Autodesk Inventor part; units mm, degrees
ref_plane "YZ Plane" through (0, 0, 0) normal (1, 0, 0) x (0, 1, 0)
ref_plane "XZ Plane" through (0, 0, 0) normal (0, 1, 0) x (-1, 0, 0)
ref_plane "XY Plane" through (0, 0, 0) normal (0, 0, 1) x (1, 0, 0)
ref_plane "Work Plane1" through (0, 0, 0) normal (0, 0, 1) x (1, 0, 0)
sketch "Sketch1" plane through (0, 0, 0) normal (0, 0, 1) x (1, 0, 0)
  circle A0 centre (11.7233, 46.6483) radius 2.132
  circle A1 centre (20.0025, 56.1975) radius 2.132
  circle A2 centre (32.7025, 56.1975) radius 2.132
  circle A3 centre (45.4025, 56.1975) radius 2.132
  circle A4 centre (58.1025, 56.1975) radius 2.132
  circle A5 centre (-58.7375, 17.4625) radius 2.132
  circle A6 centre (-46.6483, 46.6483) radius 2.132
  circle A7 centre (-17.4625, 58.7375) radius 2.132
  circle A8 centre (11.7233, 46.6483) radius 2.132
  circle A9 centre (23.8125, 17.4625) radius 2.132
  circle A10 centre (11.7233, -11.7233) radius 2.132
  circle A11 centre (-17.4625, -23.8125) radius 2.132
  circle A12 centre (-46.6483, -11.7233) radius 2.132
  circle A13 centre (-56.1975, -32.7025) radius 2.132
  circle A14 centre (-56.1975, -45.4025) radius 2.132
  circle A15 centre (-56.1975, -58.1025) radius 2.132
  circle A16 centre (-56.1975, -20.0025) radius 2.132
  circle A17 centre (-17.4625, 17.4625) radius 38.1
  circle A18 centre (-17.4625, 17.4625) radius 38.3
  circle A19 centre (-17.4625, 17.4625) radius 45.72
  circle A20 centre (-17.4625, 17.4625) radius 32.55
  line L0 (9.485, -18.7266) -> (-48.7269, -62.0728)
  arc A21 (9.485, -18.7266) -> (18.7266, -9.485) centre (-17.4625, 17.4625) ccw
  line L1 (62.0728, 48.7269) -> (18.7266, -9.485)
  arc A22 (62.0728, 48.7269) -> (62.5825, 50.2648) centre (60.0075, 50.2648) ccw
  line L2 (62.5825, 60.0075) -> (62.5825, 50.2648)
  arc A23 (62.5825, 60.0075) -> (60.0075, 62.5825) centre (60.0075, 60.0075) ccw
  line L3 (-17.4625, 62.5825) -> (60.0075, 62.5825)
  arc A24 (-17.4625, 62.5825) -> (-62.5825, 17.4625) centre (-17.4625, 17.4625) ccw
  line L4 (-62.5825, -60.0075) -> (-62.5825, 17.4625)
  arc A25 (-62.5825, -60.0075) -> (-60.0075, -62.5825) centre (-60.0075, -60.0075) ccw
  line L5 (-50.2648, -62.5825) -> (-60.0075, -62.5825)
  arc A26 (-50.2648, -62.5825) -> (-48.7269, -62.0728) centre (-50.2648, -60.0075) ccw
  arc A27 (-46.4955, -21.6632) -> (-38.635, -17.6063) centre (-46.6483, -11.7233) ccw
  arc A28 (-33.9418, -16.445) -> (-38.635, -17.6063) centre (-35.592, -19.8403) ccw
  arc A29 (-33.9418, -16.445) -> (-29.7861, -18.1664) centre (-17.4625, 17.4625) ccw
  arc A30 (-27.2887, -22.3061) -> (-29.7861, -18.1664) centre (-31.0201, -21.734) ccw
  arc A31 (-27.2887, -22.3061) -> (-26.8535, -27.0731) centre (-17.4625, -23.8125) ccw
  arc A32 (-28.1651, -31.3391) -> (-26.8535, -27.0731) centre (-30.4197, -28.3113) ccw
  line L6 (-44.1828, -43.2664) -> (-28.1651, -31.3391)
  arc A33 (-50.2124, -40.2386) -> (-44.1828, -43.2664) centre (-46.4374, -40.2386) ccw
  line L7 (-50.2124, -25.4377) -> (-50.2124, -40.2386)
  arc A34 (-46.4955, -21.6632) -> (-50.2124, -25.4377) centre (-46.4374, -25.4377) ccw
  line L8 (40.2386, 50.2124) -> (25.4377, 50.2124)
  arc A35 (43.2664, 44.1828) -> (40.2386, 50.2124) centre (40.2386, 46.4374) ccw
  line L9 (31.3391, 28.1651) -> (43.2664, 44.1828)
  arc A36 (27.0731, 26.8535) -> (31.3391, 28.1651) centre (28.3113, 30.4197) ccw
  arc A37 (27.0731, 26.8535) -> (22.3061, 27.2887) centre (23.8125, 17.4625) ccw
  arc A38 (18.1664, 29.7861) -> (22.3061, 27.2887) centre (21.734, 31.0201) ccw
  arc A39 (18.1664, 29.7861) -> (16.445, 33.9418) centre (-17.4625, 17.4625) ccw
  arc A40 (17.6063, 38.635) -> (16.445, 33.9418) centre (19.8403, 35.592) ccw
  arc A41 (17.6063, 38.635) -> (21.6632, 46.4955) centre (11.7233, 46.6483) ccw
  arc A42 (25.4377, 50.2124) -> (21.6632, 46.4955) centre (25.4377, 46.4374) ccw
  point P0 (0, 0)
  dimension "d0" = 0.2
extrude "Extrusion1" add sketch "Sketch1" along normal blind 7.6 contours A38 A37 A36 A19 L1 A21 L0 A32 A31 A30 A18 | A18 A40 A41 A19 A36 A37 A38 | A30 A31 A32 A19 A27 A28 A18 | A18 A28 A27 A19 L4 A24 L3 A41 A40 | L3 A24 L4 A19 | L0 A21 L1 A19
properties part number "upper_plate"
Build history of the part. All positions in model axes, mm. Coordinates: 2 decimals unless noted, no trailing zeros. Order: outer loops, then holes, each group sorted by start corner. A loop starts at its lowest first (then second) coordinate and runs counter-clockwise, first axis right, second up. Notation, with made-up numbers: (60, 29) -> (105, 29) arc R15 ccw to (105, 44) -> close; hole circle Ø2 at (55, -27). An arc over 180 degrees is marked (long way). Answer in a Markdown table with one row per item. Add a question column.
Q1. Band-saw the part on D-D, the plane z = 4. Give the number of separate pieces and of enclosed holes in the cut face, then the cut area to 3 significant figures.
Q2. Band-saw the part on A-A, the plane x = -17. List the corners of the cut face in (y, z), then the cut area to 3 significant figures.
Q3. Band-saw the part on C-C, the plane x = -52. List the corners of the cut face in (y, z).
Q4. Drop flat-ended pins along their axis: pin 1 (1.5 mm diameter, centred on x = -21, z = 4.5, fed in from +Y); pin 2 (1 mm diameter, centred on x = 5, z = 3, fed in from -Y); pin 3 (3 mm diameter, centred on x = -17.5, z = 5, fed in from +Y). Give the stop position or say it passes through.
Q5. Mould opens along X. For faces 1 (the face through (-48, 45, 4)), 2 (the face through (-51.16, -13.44, 3.75)), 3 (the face through (6, 48, 7.6)) say: +X half, -X half, draft (parallel to the pull), parting line (faces both ways), or undercut.
Q6. Wall check: line 1 along X through (y, z) = (16.5, 6.75); line 2 along Y through (x, z) = (-59, 0.5); line 3 along X through (y, z) = (41.5, 4.25). Give the ranges that are in metal, low to high. Write a range as [from, to].
Q7. Band-saw the part on B-B, the plane y = 7. List the corners of the cut face in (x, z), then the cut area to 3 significant figures.
Answers follow:
| question | item | result |
|---|---|---|
| 1 | separate pieces | 1 |
| 1 | enclosed holes | 9 |
| 1 | area | 1,840 mm^2 |
| 2 | outline | (-28.26, 0) -> (-25.89, 0) -> (-25.89, 7.6) -> (-28.26, 7.6) -> close; (-21.73, 0) -> (-20.83, 0) -> (-20.83, 7.6) -> (-21.73, 7.6) -> close; (55.76, 0) -> (56.66, 0) -> (56.66, 7.6) -> (55.76, 7.6) -> close; (60.82, 0) -> (63.18, 0) -> (63.18, 7.6) -> (60.82, 7.6) -> close |
| 2 | area | 49.5 mm^2 |
| 3 | outline | (-12.5, 0) -> (0.91, 0) -> (0.91, 7.6) -> (-12.5, 7.6) -> close; (34.02, 0) -> (47.42, 0) -> (47.42, 7.6) -> (34.02, 7.6) -> close |
| 4 | pin 1 | y = 63.1 |
| 4 | pin 2 | y = -22.64 |
| 4 | pin 3 | y = 63.18 |
| 5 | face 1 | undercut |
| 5 | face 2 | parting line |
| 5 | face 3 | draft |
| 6 | line 1 | [-63.17, -60.64], [-56.84, -55.75], [20.83, 21.91], [25.71, 28.25] |
| 6 | line 2 | [-1.64, 15.35], [19.58, 36.57] |
| 6 | line 3 | [-56.35, -47.28], [12.36, 21.43] |
| 7 | outline | (-61.97, 0) -> (-54.31, 0) -> (-54.31, 7.6) -> (-61.97, 7.6) -> close; (19.38, 0) -> (27.04, 0) -> (27.04, 7.6) -> (19.38, 7.6) -> close |
| 7 | area | 116 mm^2 |
